Geometry check sheet. Reference: the model listing, model coordinates, mm. A direction names the side the tool comes from. Coordinates: 2 decimals unless noted, no trailing zeros. Write each loop counter-clockwise with the first axis right and the second up, starting at its lowest first coordinate (ties: lowest second). Pieces come first, ordered by that corner, then holes.
from build123d import *

# Parameters (mm, degrees)
BOSS_EXTRUDE1_DEPTH      = 37.465
BOSS_EXTRUDE1_DEPTH_BACK = 37.465
FILLET1_R                = 1.27
SKETCH2_R                = 1.5875
CUT_EXTRUDE1_DEPTH       = 58.080672394


with BuildPart() as part:
    # Sketch1 → Boss-Extrude1 (new, two sides: drawn at the far end of the back side and taken through both)
    with BuildSketch(Plane(origin=(0, 0, 0), x_dir=(0, 0, -1), z_dir=(1, 0, 0)).offset(-BOSS_EXTRUDE1_DEPTH_BACK)):
        with BuildLine():
            Line((-25.175589489, 0), (13.918974615, 0))
            ThreePointArc((13.918974615, 0), (15.909788429, 0.824622082), (16.734410511, 2.815435896))
            Line((16.734410511, 2.815435896), (16.734410511, 9.906))
            Line((16.734410511, 9.906), (15.146910511, 9.906))
            Line((15.146910511, 9.906), (15.146910511, 2.815435896))
            ThreePointArc((15.146910511, 2.815435896), (14.787256414, 1.947154097), (13.918974615, 1.5875))
            Line((13.918974615, 1.5875), (-25.175589489, 1.5875))
            Line((-25.175589489, 1.5875), (-25.175589489, 0))
        make_face()
    extrude(amount=BOSS_EXTRUDE1_DEPTH + BOSS_EXTRUDE1_DEPTH_BACK)

    # Fillet1
    fillet1_edges = [part.edges().sort_by_distance(p)[0] for p in [
        (-37.465, 9.906, -15.940660511),
        (37.465, 0.79375, 25.175589489),
        (37.465, 9.906, -15.940660511),
        (-37.465, 0.79375, 25.175589489),
    ]]
    fillet(fillet1_edges, radius=FILLET1_R)

    # Sketch2 → Cut-Extrude1 (cut, through all)
    with BuildSketch(Plane(origin=(0, 0, -16.734410511), x_dir=(-1, 0, 0), z_dir=(0, 0, -1))):
        with Locations((-26.9875, 6.360717948)):
            Circle(SKETCH2_R)
        with Locations((-16.1925, 6.360717948)):
            Circle(SKETCH2_R)
        with Locations((-5.3975, 6.360717948)):
            Circle(SKETCH2_R)
        with Locations((5.3975, 6.360717948)):
            Circle(SKETCH2_R)
        with Locations((16.1925, 6.360717948)):
            Circle(SKETCH2_R)
        with Locations((26.9875, 6.360717948)):
            Circle(SKETCH2_R)
    extrude(amount=-CUT_EXTRUDE1_DEPTH, mode=Mode.SUBTRACT)


solid = part.part
1. Sectioned sample at C-C, the plane z = 14.5. Record the boundary of the cut face in (x, y) (1 decimal).
Computed values:
outline: (-37.5, 0) - (37.5, 0) - (37.5, 1.6) - (-37.5, 1.6) - close
2. Sectioned sample at B-B, the plane x = 11. Record the boundary of the cut face in (y, z), and give its area (3 significant figures).
Computed values:
outline: (0, -13.92) arc R2.82 ccw to (2.82, -16.73) - (9.91, -16.73) - (9.91, -15.15) - (2.82, -15.15) arc R1.23 cw to (1.59, -13.92) - (1.59, 25.18) - (0, 25.18) - close
area: 78.4 mm2
3. Thickness scan on line 1 along Z through (x, y) = (-5.5, 9.5); line 2 along Y through (x, z) = (12, 0); line 3 along Z through (x, y) = (28, 1.25). Record the ranges inside material, lowest first.
Computed values:
line 1: z = -16.73 to -15.15
line 2: y = 0 to 1.59
line 3: z = -16.26 to 25.18
4. Draft check along X on faces 3 (the cylindrical face through (6.657, 5.395, -15.952)), 4 (the flat face through (-1, 1.588, 5)), 5 (the flat face through (-37.465, 1, 1)), 6 (the cylindrical face through (28.573, 6.431, -15.952)). Enter one of: released by +X, released by -X, zero draft, split by the parting line, or undercut.
Computed values:
face 3: undercut
face 4: zero draft
face 5: released by -X
face 6: undercut
5. Access from +Z, -Z, +X, -X, +Y, -Y to the whole of each face (thin tool, end or side, straight path). Record for faces 1 (the flat face through (-1, 9.906, -16)), 2 (the flat face through (-1, 6, -15.147)).
Computed values:
face 1: +Z, -Z, +X, -X, +Y
face 2: +Z, +X, -X, +Y
6. Sectioned sample at A-A, the plane x = -27.5. Record the boundary of the cut face in (y, z).
Computed values:
outline: (0, -13.92) arc R2.82 ccw to (2.82, -16.73) - (4.86, -16.73) - (4.86, -15.15) - (2.82, -15.15) arc R1.23 cw to (1.59, -13.92) - (1.59, 25.18) - (0, 25.18) - close; (7.86, -16.73) - (9.91, -16.73) - (9.91, -15.15) - (7.86, -15.15) - close
7. Gauge pin test, flat ends, axial feed: pin 1 Ø1.9 at (x, y) = (-26.99, 6.36) entering from -Z; pin 2 Ø1 at (y, z) = (2, -4) entering from -X (3 decimals); pin 3 Ø4 at (x, y) = (26.99, 6.36) entering from +Z. Record the tip position at first contact, or that the pin passes through.
Computed values:
pin 1: passes through
pin 2: stops at x = -37.465
pin 3: stops at z = -15.15
